Read the model definition and answer for the solid it produces. Units are mm, in the model's axes. Face numbers are marked on the shaded views. A direction names the side the tool comes from. Round coordinates to 2 decimals unless told otherwise and drop trailing zeros. Write each loop counter-clockwise with the first axis right and the second up, starting at its lowest first coordinate (ties: lowest second). Pieces come first, ordered by that corner, then holes. Notation, with made-up numbers: (37, -24) -> (84, -24) arc R24 cw to (84, 13) -> close; hole circle Ø3 at (29, 65). An arc over 180 degrees is marked (long way). Return JSON: item names as keys, results as strings. Group by question number.
(1) Given pin 1 (1 mm diameter, centred on x = 7, y = -8.5, fed in from -Z); pin 2 (18.5 mm diameter, centred on x = 8, y = -27.5, fed in from +Z); pin 3 (6 mm diameter, centred on y = -31, z = 16.5, fed in from +X), each flat-ended and moving along its own axis, determine where each tip first touches the part or whether it passes through.
(2) Straight lines are drawn through the part: line 1 (X direction, y = -19, z = 46); line 2 (Z direction, x = -20.5, y = -35); line 3 (Z direction, x = 13.5, y = -10.5). For each, find the intervals that lie inside material, in ascending order.
(3) For the marked faces 1, 2 and 3, determine the directions among +Z, -Z, +X, -X, +Y, -Y from which every point of the face is accessible in a straight line to the end or side of a thin tool.
(4) A cutting plane is placed at B-B on x = -15. Give the vertices of the cut face in (y, z), then the cut area to 3 significant figures.
(5) A cutting plane is placed at A-A on y = -33.5. Give the vertices of the cut face in (x, z).
(6) A cutting plane is placed at C-C on z = 47.5. Give the vertices of the cut face in (x, y).
```python
from build123d import *

# Parameters (mm, degrees)
F1_DEPTH = 37.338


with BuildPart() as f1:
    # F0 (on Front) → F1 (new body)
    with BuildSketch(Plane.XZ):
        Polygon((36.141854, 44.383232), (71.51109, 44.383232), (71.51109, 64.299881), (53.826472, 64.299881), (36.141854, 64.299881), align=None)
        Polygon((-74.336521, 0), (0, 0), (0, 25.665386), (-26.011834, 25.665386), (-74.336521, 25.665386), align=None)
        Polygon((-26.011834, 25.665386), (0, 25.665386), (71.51109, 25.665386), (71.51109, 44.383232), (36.141854, 44.383232), (-26.011834, 44.383232), align=None)
    extrude(amount=F1_DEPTH)


solid = f1.part
```
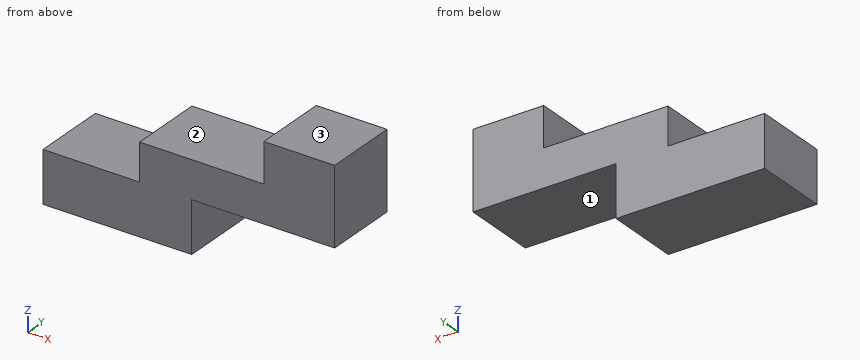
Checks:
{
 "1": {"pin 1": "stops at z = 25.67", "pin 2": "stops at z = 44.38", "pin 3": "stops at x = 0"},
 "2": {"line 1": "x = 36.14 to 71.51", "line 2": "z = 0 to 44.38", "line 3": "z = 25.67 to 44.38"},
 "3": {"face 1": "-Z, +X, +Y, -Y", "face 2": "+Z, -X, +Y, -Y", "face 3": "+Z, +X, -X, +Y, -Y"},
 "4": {"outline": "(-37.34, 0) -> (0, 0) -> (0, 44.38) -> (-37.34, 44.38) -> close", "area": "1,660 mm^2"},
 "5": {"outline": "(-74.34, 0) -> (0, 0) -> (0, 25.67) -> (71.51, 25.67) -> (71.51, 64.3) -> (36.14, 64.3) -> (36.14, 44.38) -> (-26.01, 44.38) -> (-26.01, 25.67) -> (-74.34, 25.67) -> close"},
 "6": {"outline": "(36.14, -37.34) -> (71.51, -37.34) -> (71.51, 0) -> (36.14, 0) -> close"}
}
